For this review, take the finished solid that the model builds, in its own axes (mm). Round coordinates to 2 decimals unless told otherwise and drop trailing zeros. One line per item, written item: value.
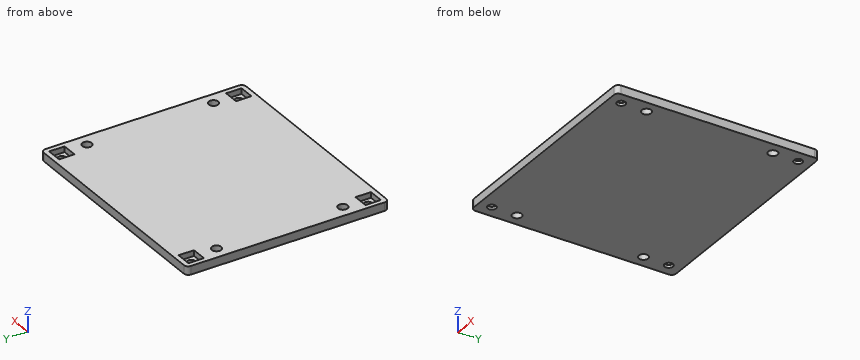
```python
from build123d import *

# Parameters (mm, degrees)
MODEL_R                 = 1.5
MODEL_R_2               = 1.7
SALIENTE_EXTRUIR1_DEPTH = 3
CROQUIS2_W              = 5.5
CROQUIS2_H              = 5.5
CORTAR_EXTRUIR1_DEPTH   = 2


with BuildPart() as part:
    # Model → Saliente-Extruir1 (new body)
    with BuildSketch(Plane.XY):
        with BuildLine():
            Line((85.482701858, 227.246277544), (7.478092, 227.246277544))
            ThreePointArc((7.478092, 227.246277544), (6.417431828, 227.685617372), (5.978092, 228.746277544))
            Line((5.978092, 228.746277544), (5.978092, 297.748681778))
            ThreePointArc((5.978092, 297.748681778), (6.417431828, 298.80934195), (7.478092, 299.248681778))
            Line((7.478092, 299.248681778), (85.482701858, 299.248681778))
            ThreePointArc((85.482701858, 299.248681778), (86.54336203, 298.80934195), (86.982701858, 297.748681778))
            Line((86.982701858, 297.748681778), (86.982701858, 228.746277544))
            ThreePointArc((86.982701858, 228.746277544), (86.54336203, 227.685617372), (85.482701858, 227.246277544))
        make_face()
        with Locations((82.48303636, 294.748681778)):
            Circle(MODEL_R, mode=Mode.SUBTRACT)
        with Locations((10.478092, 231.745943042)):
            Circle(MODEL_R, mode=Mode.SUBTRACT)
        with Locations((82.48303636, 231.745943042)):
            Circle(MODEL_R, mode=Mode.SUBTRACT)
        with Locations((10.478092, 294.748681778)):
            Circle(MODEL_R, mode=Mode.SUBTRACT)
        with Locations((10.478092, 240.74560854)):
            Circle(MODEL_R_2, mode=Mode.SUBTRACT)
        with Locations((10.478092, 285.74901628)):
            Circle(MODEL_R_2, mode=Mode.SUBTRACT)
        with Locations((82.48303636, 240.74560854)):
            Circle(MODEL_R_2, mode=Mode.SUBTRACT)
        with Locations((82.48303636, 285.74901628)):
            Circle(MODEL_R_2, mode=Mode.SUBTRACT)
    extrude(amount=SALIENTE_EXTRUIR1_DEPTH)

    # Croquis2 → Cortar-Extruir1 (cut)
    with BuildSketch(Plane.XY.offset(3)):
        with Locations((10.478092, 294.748681778)):
            Rectangle(CROQUIS2_W, CROQUIS2_H)
        with Locations((82.48303636, 294.748681778)):
            Rectangle(CROQUIS2_W, CROQUIS2_H)
        with Locations((10.478092, 231.745943042)):
            Rectangle(CROQUIS2_W, CROQUIS2_H)
        with Locations((82.48303636, 231.745943042)):
            Rectangle(CROQUIS2_W, CROQUIS2_H)
    extrude(amount=-CORTAR_EXTRUIR1_DEPTH, mode=Mode.SUBTRACT)


solid = part.part
```
Item 1: For P1, Ø5, axis at x = 10.48, y = 231.75, coming from the +Z side; P2, Ø2, axis at x = 82.48, y = 240.75, coming from the +Z side, all flat-tipped, find the tip position at first contact; note any pin that passes through.
Returned:
P1: z = 1
P2: through
Item 2: Take a section at A-A (z = 2.5). Count the separate pieces of the cut face and the enclosed holes in it, plus the area to 3 significant figures.
Returned:
separate pieces: 1
enclosed holes: 8
area: 5,670 mm^2
Item 3: Wall thickness on line 1 (X direction, y = 232.5, z = 2.9); line 2 (X direction, y = 294, z = 0.9); line 3 (Y direction, x = 83.5, z = 1.35): over which ranges is each line inside the solid? List them lowest first.
Returned:
line 1: 5.98 to 7.73, 13.23 to 79.73, 85.23 to 86.98
line 2: 5.98 to 9.18, 11.78 to 81.18, 83.78 to 86.98
line 3: 227.25 to 229, 234.5 to 239.38, 242.11 to 284.39, 287.11 to 292, 297.5 to 299.25
